Verification items for this drawing (mm, ordinates from the low corner). A direction names the side the tool comes from. Round coordinates to 2 decimals unless told otherwise and drop trailing zeros. Loops run counter-clockwise (first coordinate to the right, second up) from the corner with the lowest first, then second, coordinate; pieces in that order, holes last. Notation, with made-up numbers: M 70.5,-40 L 126.5,-40 A17 cw 126.5,-23 Z; hole C 47,26.25 d7. An arc over 180 degrees is marked long. Write item = value, one per line.
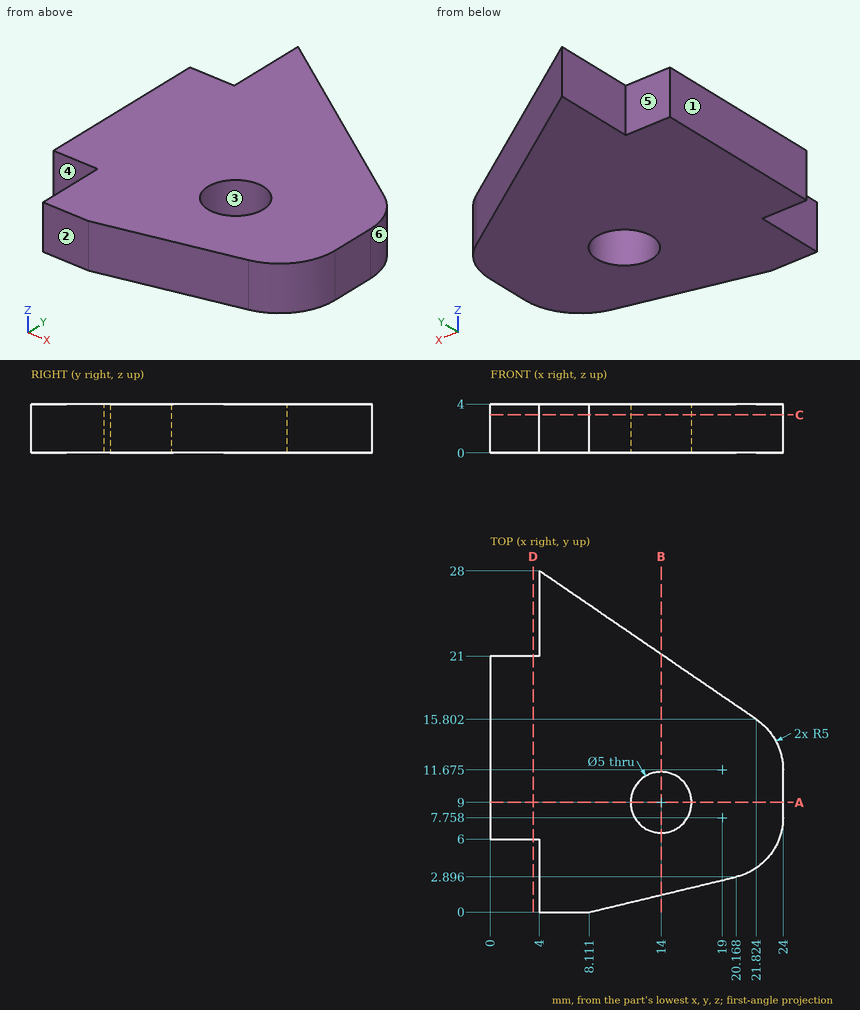
(1) Release check for a two-part mould opening along Y. For the marked faces 1, 2 and 3 record: released by +Y, released by -Y, zero draft, split by the parting line, or undercut.
Result set:
face_1 = zero draft
face_2 = released by -Y
face_3 = undercut
(2) Sectioned sample at A-A on y = 9. Record the cut outline in (x, z), then the cut area to 3 significant figures.
Result set:
outline = M 0,0 L 11.5,0 L 11.5,4 L 0,4 Z; M 16.5,0 L 24,0 L 24,4 L 16.5,4 Z
area = 76.0 mm2
(3) Sectioned sample at D-D on x = 3.5. Record the cut outline in (y, z), then the cut area to 3 significant figures.
Result set:
outline = M 6,0 L 21,0 L 21,4 L 6,4 Z
area = 60.0 mm2
(4) Depth check by flat-ended pin: pin 1 Ø1.2 at (x, z) = (2, 2.5) entering from +Y; pin 2 Ø4.5 at (x, y) = (14, 9) entering from +Z; pin 3 Ø2 at (x, z) = (11.5, 1) entering from +Y. Enter the tip coordinate at first touch or a pass-through.
Result set:
pin_1 = 21
pin_2 = through
pin_3 = 23.55
(5) Tool access check on the marked faces 4, 5 and 6. Record the directions out of +Z, -Z, +X, -X, +Y, -Y that give a thin tool (end or side, any length) a straight path to the whole face; none if there is none.
Result set:
face_4 = +Z, -Z, -X, -Y
face_5 = +Z, -Z, -X, +Y
face_6 = +Z, -Z, +X, +Y
(6) Sectioned sample at B-B on x = 14. Record the cut outline in (y, z) (1 decimal).
Result set:
outline = M 1.4,0 L 6.5,0 L 6.5,4 L 1.4,4 Z; M 11.5,0 L 21.2,0 L 21.2,4 L 11.5,4 Z
(7) Material ranges on line 1 along Y through (x, z) = (14, 1.05) (1 decimal); line 2 along X through (y, z) = (11.25, 1.7) (1 decimal); line 3 along Y through (x, z) = (2, 1.65), recorded low to high. Write a range as from..to.
Result set:
line_1 = 1.4..6.5, 11.5..21.2
line_2 = 0..12.9, 15.1..24
line_3 = 6..21
(8) Sectioned sample at C-C on z = 3.1. Record the cut outline in (x, y) (1 decimal), then the cut area to 3 significant figures.
Result set:
outline = M 0,6 L 4,6 L 4,0 L 8.1,0 L 20.2,2.9 A5 ccw 24,7.8 L 24,11.7 A5 ccw 21.8,15.8 L 4,28 L 4,21 L 0,21 Z; hole C 14,9 d5
area = 429 mm2
